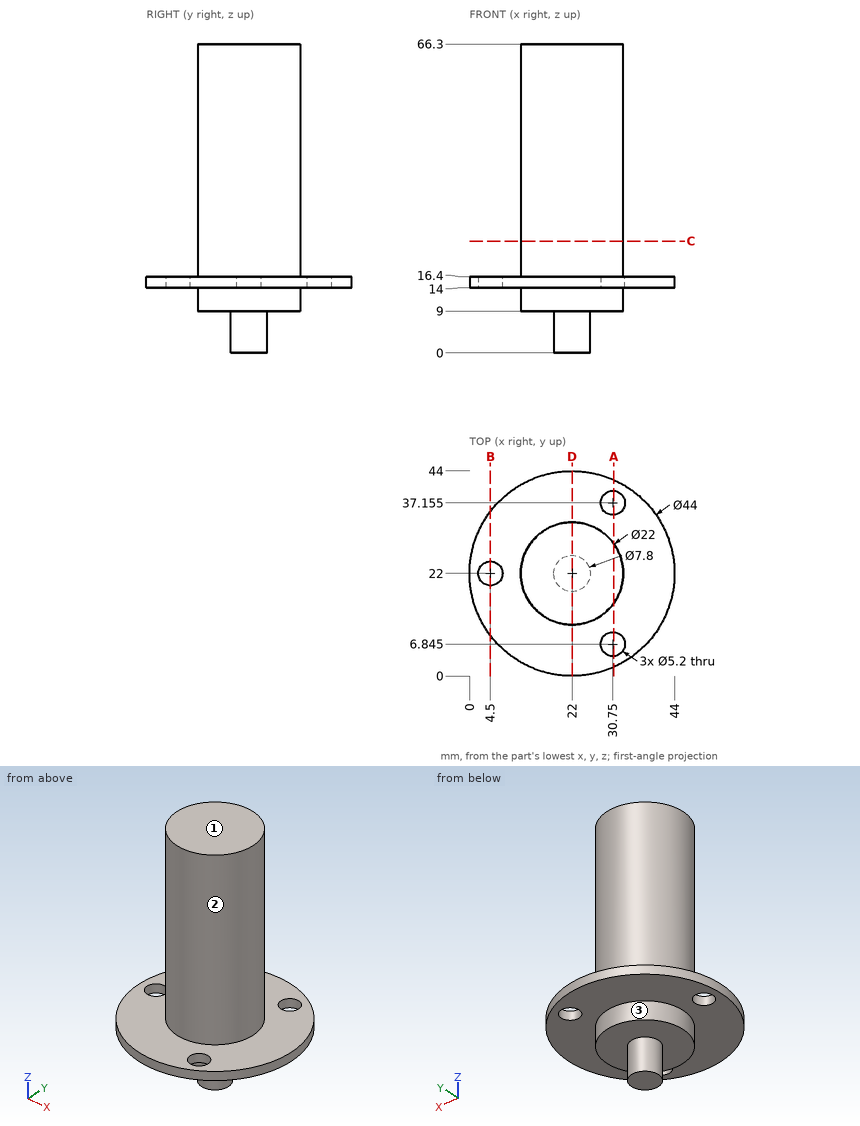
Check sheet for the drawn part. Datum: minimum x, y, z corner. Units: mm. A direction names the side the tool comes from. Coordinates: 2 decimals unless noted, no trailing zeros. Loops run counter-clockwise (first coordinate to the right, second up) from the corner with the lowest first, then second, coordinate; pieces in that order, holes last. Notation, with made-up numbers: (47.25, -17.5) - (80.25, -17.5) arc R17 ccw to (80.25, 1.5) - close; hole circle Ø9 at (51.5, 52). An arc over 180 degrees is marked (long way). Put each result on its own line as item: value.
Item 1: Gauge pin test, flat ends, axial feed: pin 1 Ø1 at (y, z) = (30.5, 57.5) entering from -X; pin 2 Ø10 at (x, z) = (38.5, 24.5) entering from +Y; pin 3 Ø10 at (y, z) = (32.5, 22) entering from +X; pin 4 Ø6 at (x, y) = (31, 5) entering from -Z. Record the tip position at first contact, or that the pin passes through.
Conclusion:
pin 1: stops at x = 14.45
pin 2: passes through
pin 3: stops at x = 31.53
pin 4: stops at z = 14
Item 2: Set-up check for the marked faces 1, 2 and 3: record each of +Z, -Z, +X, -X, +Y, -Y from which the full face is reachable in a straight line by a thin tool's end or side.
Conclusion:
face 1: +Z, +X, -X, +Y, -Y
face 2: +Z
face 3: -Z
Item 3: Section check C-C (z = 24). Enter the section's corners in (x, y).
Conclusion:
outline: circle Ø22 at (22, 22)
Item 4: Scan lines: line 1 along Z through (x, y) = (10.5, 35.5); line 2 along Y through (x, z) = (30.75, 15.15) (1 decimal); line 3 along Z through (x, y) = (29.5, 25.5). Record each from-to range of solid material in increasing order.
Conclusion:
line 1: z = 14 to 16.4
line 2: y = 1.8 to 4.2, 9.4 to 34.6, 39.8 to 42.2
line 3: z = 9 to 66.3
Item 5: Section check D-D (x = 22). Enter the section's corners in (y, z).
Conclusion:
outline: (0, 14) - (11, 14) - (11, 9) - (18.1, 9) - (18.1, 0) - (25.9, 0) - (25.9, 9) - (33, 9) - (33, 14) - (44, 14) - (44, 16.4) - (33, 16.4) - (33, 66.3) - (11, 66.3) - (11, 16.4) - (0, 16.4) - close
Item 6: Section check A-A (x = 31). Enter the section's corners in (y, z) (1 decimal), then the cut area to 3 significant figures.
Conclusion:
outline: (1.9, 14) - (4.3, 14) - (4.3, 16.4) - (1.9, 16.4) - close; (9.4, 14) - (15.7, 14) - (15.7, 9) - (28.3, 9) - (28.3, 14) - (34.6, 14) - (34.6, 16.4) - (28.3, 16.4) - (28.3, 66.3) - (15.7, 66.3) - (15.7, 16.4) - (9.4, 16.4) - close; (39.7, 14) - (42.1, 14) - (42.1, 16.4) - (39.7, 16.4) - close
area: 766 mm2
Item 7: Section check B-B (x = 4.5). Enter the section's corners in (y, z).
Conclusion:
outline: (8.67, 14) - (19.4, 14) - (19.4, 16.4) - (8.67, 16.4) - close; (24.6, 14) - (35.33, 14) - (35.33, 16.4) - (24.6, 16.4) - close
